Can you work these out from the model? Positions are in its coordinate system, mm. A direction names the side the tool comes from. Give positions to 0.01 mm unless a question says otherwise; leave off trailing zeros. Write each loop counter-clockwise with the first axis right and the second up, starting at its lowest first coordinate (ties: lowest second). Pieces come first, ordered by that corner, then holes.
```python
from build123d import *

# Parameters (mm, degrees)
SKETCH1_R           = 3.556
SKETCH1_R_2         = 1.9812
SKETCH1_W           = 63.5
SKETCH1_H           = 3.175
BOSS_EXTRUDE1_DEPTH = 3.175


with BuildPart() as part:
    # Sketch1 → Boss-Extrude1 (new body)
    with BuildSketch(Plane(origin=(0, 0, 0), x_dir=(0, 0, -1), z_dir=(1, 0, 0))):
        Polygon((-66.675, 28.575), (-31.75, 28.575), (-31.75, 32.385), (31.75, 32.385), (31.75, 28.575), (66.675, 28.575), (66.675, 15.875), (70.485, 15.875), (70.485, -15.875), (66.675, -15.875), (66.675, -34.29), (-66.675, -34.29), (-66.675, -15.875), (-70.485, -15.875), (-70.485, 15.875), (-66.675, 15.875), align=None)
        with Locations((4.445, -13.335)):
            Circle(SKETCH1_R, mode=Mode.SUBTRACT)
        with Locations((-53.975, -23.6347)):
            Circle(SKETCH1_R_2, mode=Mode.SUBTRACT)
        with Locations((0, -30.1625)):
            Rectangle(SKETCH1_W, SKETCH1_H, mode=Mode.SUBTRACT)
    extrude(amount=BOSS_EXTRUDE1_DEPTH)


solid = part.part
```
1) Please list where these lines run through material, in increasing order: L1, parallel to Y at x = 2.45, z = -17.5 (3 decimals); L2, parallel to Y at x = 2, z = -65 (3 decimals); L3, parallel to Z at x = 1.55, y = -29.5 (3 decimals).
Values follow:
L1: y = -34.29 to -31.75, -28.575 to 32.385
L2: y = -34.29 to 28.575
L3: z = -66.675 to -31.75, 31.75 to 66.675
2) For pin 1 Ø11.5 at (y, z) = (-13.335, -4.445) entering from +X (3 decimals); pin 2 Ø1.6 at (x, z) = (1.5, 69.5) entering from -Y (3 decimals); pin 3 Ø2.5 at (y, z) = (-23.63, 53.98) entering from +X; pin 4 Ø1 at (x, y) = (2, 19) entering from -Z (3 decimals), each with a flat end and sliding along its axis, tell me the tip position at first contact or that it passes through.
Values follow:
pin 1: stops at x = 3.175
pin 2: stops at y = -15.875
pin 3: passes through
pin 4: stops at z = -66.675
3) Suppose I cut it at C-C on x = 2.1. Write out the boundary of the cut face in (y, z) (3 decimals).
Values follow:
outline: (-34.29, -66.675) - (-15.875, -66.675) - (-15.875, -70.485) - (15.875, -70.485) - (15.875, -66.675) - (28.575, -66.675) - (28.575, -31.75) - (32.385, -31.75) - (32.385, 31.75) - (28.575, 31.75) - (28.575, 66.675) - (15.875, 66.675) - (15.875, 70.485) - (-15.875, 70.485) - (-15.875, 66.675) - (-34.29, 66.675) - close; hole (-31.75, -31.75) - (-28.575, -31.75) - (-28.575, 31.75) - (-31.75, 31.75) - close; hole circle Ø3.962 at (-23.635, 53.975); hole circle Ø7.112 at (-13.335, -4.445)
4) Suppose I cut it at B-B on y = -30. Write out the boundary of the cut face in (x, z) (3 decimals).
Values follow:
outline: (0, -66.675) - (3.175, -66.675) - (3.175, -31.75) - (0, -31.75) - close; (0, 31.75) - (3.175, 31.75) - (3.175, 66.675) - (0, 66.675) - close
5) For faces 5 (the face through (2, -25, -66.675)), 6 (the face through (2, -25, 66.675)), 7 (the face through (2, 28.575, 49)), which set-ups out of +Z, -Z, +X, -X, +Y, -Y let a thin tool reach every point of the face, with its end or its side?
Values follow:
face 5: -Z, +X, -X, -Y
face 6: +Z, +X, -X, -Y
face 7: +Z, +X, -X, +Y
6) If we mould it in two halves opening along Y, with no side actions, what happens to faces 1 (the face through (2, 28.575, -49)), 2 (the face through (2, 22, 66.675)), 3 (the face through (2, -34.29, -1)), 4 (the face through (2, -28.575, 0))? For each: +Y half, -Y half, draft (parallel to the pull), parting line (faces both ways), or undercut.
Values follow:
face 1: +Y half
face 2: draft
face 3: -Y half
face 4: undercut
7) Suppose I cut it at D-D on y = 27. Write out the boundary of the cut face in (x, z) (3 decimals), plus the area to 3 significant figures.
Values follow:
outline: (0, -66.675) - (3.175, -66.675) - (3.175, 66.675) - (0, 66.675) - close
area: 423 mm2
8) Suppose I cut it at A-A on z = -13.5. Write out the boundary of the cut face in (x, y) (3 decimals).
Values follow:
outline: (0, -34.29) - (3.175, -34.29) - (3.175, -31.75) - (0, -31.75) - close; (0, -28.575) - (3.175, -28.575) - (3.175, 32.385) - (0, 32.385) - close
